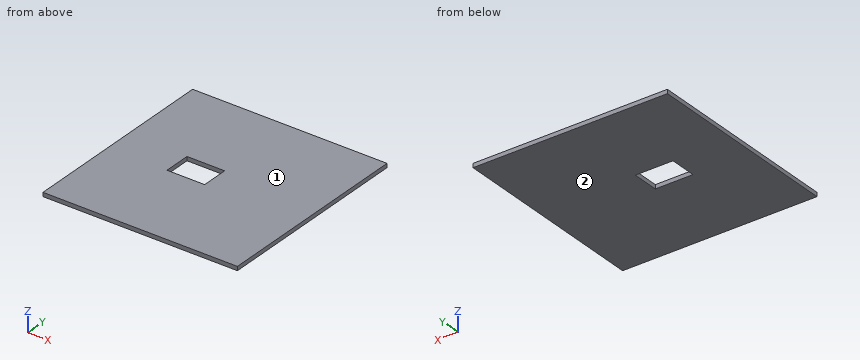
from build123d import *

# Parameters (mm, degrees)
SKETCH1_W           = 144.5
SKETCH1_H           = 149.5
BOSS_EXTRUDE1_DEPTH = 3
CUT_EXTRUDE1_REACH  = 5
SKETCH2_W           = 28
SKETCH2_H           = 20


with BuildPart() as part:
    # Sketch1 → Boss-Extrude1 (new body)
    with BuildSketch(Plane.XY):
        Rectangle(SKETCH1_W, SKETCH1_H)
    extrude(amount=BOSS_EXTRUDE1_DEPTH)

    # Sketch2 → Cut-Extrude1 (cut, up to next)
    with BuildSketch(Plane.XY.offset(3), mode=Mode.PRIVATE) as cut_extrude1_sk1:
        with Locations((-14.25, 0)):
            Rectangle(SKETCH2_W, SKETCH2_H)
    cut_extrude1_tool1 = extrude(cut_extrude1_sk1.sketch, amount=-CUT_EXTRUDE1_REACH, mode=Mode.PRIVATE) & part.part
    add(cut_extrude1_tool1.solids().sort_by_distance((-14.25, 0, 3))[0], mode=Mode.SUBTRACT)


solid = part.part
Geometry: final body of the model. Coordinates: model frame, mm. Face numbers are marked on the shaded views. Give positions to 0.01 mm unless a question says otherwise; leave off trailing zeros. Order: outer loops, then holes, each group sorted by start corner. A loop starts at its lowest first (then second) coordinate and runs counter-clockwise, first axis right, second up. Notation, with made-up numbers: (31, -35) -> (81, -35) arc R16 cw to (81, -10) -> close; hole circle Ø7 at (-25, 68.5). An arc over 180 degrees is marked (long way). Answer as a JSON object with one key per item and string values.
Q1. Material intervals for probe 1 along Y at (x, z) = (-17, 2.4), sorted ascending.
Entries:
{"probe 1": "y = -74.75 to -10, 10 to 74.75"}
Q2. Draft query along Z for the marked faces 1 and 2. Return one class per face: released by +Z, released by -Z, zero draft, split by the parting line, or undercut.
Entries:
{"face 1": "released by +Z", "face 2": "released by -Z"}
Q3. Section B-B (y = 1.5). Output: boundary loops of the cut face in (x, z).
Entries:
{"outline": "(-72.25, 0) -> (-28.25, 0) -> (-28.25, 3) -> (-72.25, 3) -> close; (-0.25, 0) -> (72.25, 0) -> (72.25, 3) -> (-0.25, 3) -> close"}
Q4. Section C-C (z = 1.35). Output: boundary loops of the cut face in (x, y).
Entries:
{"outline": "(-72.25, -74.75) -> (72.25, -74.75) -> (72.25, 74.75) -> (-72.25, 74.75) -> close; hole (-28.25, -10) -> (-0.25, -10) -> (-0.25, 10) -> (-28.25, 10) -> close"}
Q5. Section A-A (x = -13.5). Output: boundary loops of the cut face in (y, z).
Entries:
{"outline": "(-74.75, 0) -> (-10, 0) -> (-10, 3) -> (-74.75, 3) -> close; (10, 0) -> (74.75, 0) -> (74.75, 3) -> (10, 3) -> close"}
Q6. First-contact query: pin 1 (10 mm diameter, centred on x = -15.5, y = 22.5, fed in from -Z). Flat tip, straight axial feed; report the tip coordinate or a pass-through.
Entries:
{"pin 1": "stops at z = 0"}
